from build123d import *

# Parameters (mm, degrees)
BOSS_EXTRUDE1_DEPTH = 10
CUT_EXTRUDE1_DEPTH  = 7
SKETCH3_R           = 2.5
CUT_EXTRUDE2_DEPTH  = 10
CHAMFER2_SIZE       = 1
CHAMFER3_SIZE       = 1
SHELL1_START        = -7
SHELL1_OUTLINE_W    = 20
SHELL1_OUTLINE_H    = 14
SHELL1_DEPTH        = 14
CHAMFER4_SIZE       = 1


# Read off the part's stored shape, not the designer's step: Shell1
with BuildPart() as part:
    # Sketch1 → Boss-Extrude1 (new, symmetric)
    with BuildSketch(Plane.XY):
        with BuildLine():
            Line((-20, 10), (20, 10))
            ThreePointArc((20, 10), (30, 0), (20, -10))
            Line((20, -10), (-20, -10))
            ThreePointArc((-20, -10), (-30, 0), (-20, 10))
        make_face()
    extrude(amount=BOSS_EXTRUDE1_DEPTH, both=True)

    # Sketch2 → Cut-Extrude1 (cut, symmetric)
    with BuildSketch(Plane.XY):
        with BuildLine():
            Line((-20, 10), (-10, 10))
            Line((-10, 10), (-10, -10))
            Line((-10, -10), (-20, -10))
            ThreePointArc((-20, -10), (-30, 0), (-20, 10))
        make_face()
        with BuildLine():
            Line((10, -10), (20, -10))
            ThreePointArc((20, -10), (30, 0), (20, 10))
            Line((20, 10), (10, 10))
            Line((10, 10), (10, -10))
        make_face()
    extrude(amount=CUT_EXTRUDE1_DEPTH, both=True, mode=Mode.SUBTRACT)

    # Sketch3 → Cut-Extrude2 (cut, symmetric)
    with BuildSketch(Plane.XY):
        with Locations((-20, 0)):
            Circle(SKETCH3_R)
        with Locations(Location((20, 0, 0), (0, 0, 180))):
            Circle(SKETCH3_R)
    extrude(amount=CUT_EXTRUDE2_DEPTH, both=True, mode=Mode.SUBTRACT)

    # Chamfer2
    chamfer2_edges = [part.edges().sort_by_distance(p)[0] for p in [
        (-30, 0, -7),
        (-15, 10, -7),
        (-15, -10, -7),
        (-30, 0, 7),
        (-15, -10, 7),
        (-15, 10, 7),
        (30, 0, -7),
        (15, -10, -7),
        (15, 10, -7),
        (30, 0, 7),
        (15, 10, 7),
        (15, -10, 7),
    ]]
    chamfer(chamfer2_edges, length=CHAMFER2_SIZE)

    # Chamfer3
    chamfer3_edges = [part.edges().sort_by_distance(p)[0] for p in [
        (30, 0, 10),
        (0, 10, 10),
        (-30, 0, 10),
        (0, 10, -10),
        (30, 0, -10),
        (0, -10, -10),
        (-30, 0, -10),
        (0, -10, 10),
    ]]
    chamfer(chamfer3_edges, length=CHAMFER3_SIZE)

    # Shell1 outline → Shell1 (cut)
    with BuildSketch(Plane.XY.offset(SHELL1_START)):
        Rectangle(SHELL1_OUTLINE_W, SHELL1_OUTLINE_H)
    extrude(amount=SHELL1_DEPTH, mode=Mode.SUBTRACT)

    # Chamfer4
    chamfer4_edges = [part.edges().sort_by_distance(p)[0] for p in [
        (10, -10, 0),
        (10, 10, 0),
        (-10, -10, 0),
        (-10, 10, 0),
    ]]
    chamfer(chamfer4_edges, length=CHAMFER4_SIZE)


solid = part.part
Here's how the part is built. I have some questions about the finished solid (model axes, mm). A direction names the side the tool comes from. Give positions to 0.01 mm unless a question says otherwise; leave off trailing zeros. Write each loop counter-clockwise with the first axis right and the second up, starting at its lowest first coordinate (ties: lowest second). Pieces come first, ordered by that corner, then holes. Notation, with made-up numbers: (8.25, 6) -> (29.25, 6) arc R21 ccw to (29.25, 12) -> close; hole circle Ø3 at (-4, 41). An arc over 180 degrees is marked (long way). Use one line per item in the form item = value. Start each with the question number.
1. Thinking about a two-plate mould opening in Z: for faces 1 (the face through (29.2, 0.2, 9.8)), 2 (the face through (-14.6, 9.5, 7.5)), 3 (the face through (14.6, 9.5, -7.5)), 4 (the face through (-22.5, 0.1, -8.5)), which applies, +Z half, -Z half, draft (parallel to the pull), parting line (faces both ways), or undercut?
2. Imagine slicing it at B-B on z = 2.75. List the corners of the cut face in (x, y) for me.
3. Imagine slicing it at A-A on y = 0. State how many separate pieces and enclosed holes the cut face has, plus the area to 3 significant figures.
4. On a 3-axis mill with a long thin cutter (end or side, diameter ignored), from which of +Z, -Z, +X, -X, +Y, -Y can I reach the whole of each face in a straight line? I mean faces 5 (the face through (-14.4, -9.5, -7.5)), 6 (the face through (-14.6, 9.5, -7.5)), 7 (the face through (14.4, -9.5, -7.5)). Say none if no direction works.
5. Will these pins go through, and if not, where does the flat tip stop? pin 1 Ø0.6 at (y, z) = (-7.5, 0.5) entering from +X; pin 2 Ø10 at (y, z) = (-6, 5.5) entering from +X; pin 3 Ø1 at (y, z) = (-8, -0.5) entering from -X.
6. If I drill on L1, parallel to Z at x = 15.5, y = -2.5; L2, parallel to Y at x = -20, z = -8.8; L3, parallel to X at y = 1.5, z = -7.25, over which ranges is the centre line in solid material (lowest first)?
7. Imagine slicing it at C-C on x = 6. List the corners of the cut face in (y, z) for me.
Entries:
q1.face_1 = +Z half
q1.face_2 = undercut
q1.face_3 = undercut
q1.face_4 = draft
q2.outline = (-10, -9) -> (-9, -10) -> (9, -10) -> (10, -9) -> (10, -7) -> (-10, -7) -> close; (-10, 7) -> (10, 7) -> (10, 9) -> (9, 10) -> (-9, 10) -> (-10, 9) -> close
q3.separate_pieces = 6
q3.enclosed_holes = 0
q3.area = 296 mm²
q4.face_5 = -X, -Y
q4.face_6 = -X, +Y
q4.face_7 = +X, -Y
q5.pin_1 = 10
q5.pin_2 = 29.86
q5.pin_3 = -10
q6.L1 = -10 to -7, 7 to 10
q6.L2 = -10 to -2.5, 2.5 to 10
q6.L3 = -29.13 to -22, -18 to 18, 22 to 29.13
q7.outline = (-10, -9) -> (-9, -10) -> (9, -10) -> (10, -9) -> (10, 9) -> (9, 10) -> (-9, 10) -> (-10, 9) -> close; hole (-7, -7) -> (7, -7) -> (7, 7) -> (-7, 7) -> close
